Model file for the job. Use its own axes, mm. Face numbers are marked on the shaded views. A direction names the side the tool comes from. Round coordinates to 2 decimals unless told otherwise and drop trailing zeros. Loops run counter-clockwise (first coordinate to the right, second up) from the corner with the lowest first, then second, coordinate; pieces in that order, holes last. Notation, with made-up numbers: (9.5, -40) -> (45.5, -40) arc R29 ccw to (45.5, -9) -> close; hole circle Ø3 at (7, 78.5). An arc over 180 degrees is marked (long way). Use a Markdown table: item, result.
from build123d import *

# Parameters (mm, degrees)
SKETCH2_W           = 25
SKETCH2_H           = 25
BOSS_EXTRUDE1_DEPTH = 20
SKETCH3_W           = 18.8
SKETCH3_H           = 18.8
CUT_EXTRUDE1_DEPTH  = 18.8


with BuildPart() as part:
    # Sketch2 → Boss-Extrude1 (new body)
    with BuildSketch(Plane(origin=(0, 0, 0), x_dir=(1, 0, 0), z_dir=(0, 1, 0))):
        Rectangle(SKETCH2_W, SKETCH2_H)
    extrude(amount=BOSS_EXTRUDE1_DEPTH)

    # Sketch3 → Cut-Extrude1 (cut)
    with BuildSketch(Plane.XZ):
        Rectangle(SKETCH3_W, SKETCH3_H)
    extrude(amount=-CUT_EXTRUDE1_DEPTH, mode=Mode.SUBTRACT)

    # Loft1: read off the stored shape, not the designer's step
    # Loft1: loft between two sections, ruled curve by curve
    loft1_from = [
        Edge.make_bspline([(-12.5, 20, 12.5), (-11.458333333, 20, 12.5), (-10.416666667, 20, 12.5), (-8.333333333, 20, 12.5), (-7.291666667, 20, 12.5), (-5.208333333, 20, 12.5), (-4.166666667, 20, 12.5), (-2.083333333, 20, 12.5), (-1.041666667, 20, 12.5), (1.041666667, 20, 12.5), (2.083333333, 20, 12.5), (4.166666667, 20, 12.5), (5.208333333, 20, 12.5), (7.291666667, 20, 12.5), (8.333333333, 20, 12.5), (10.416666667, 20, 12.5), (11.458333333, 20, 12.5), (12.5, 20, 12.5)], [0, 0, 0, 0, 0.125, 0.125, 0.25, 0.25, 0.375, 0.375, 0.5, 0.5, 0.625, 0.625, 0.75, 0.75, 0.875, 0.875, 1, 1, 1, 1], 3),
        Edge.make_bspline([(12.5, 20, 12.5), (12.5, 20, 11.458333333), (12.5, 20, 10.416666667), (12.5, 20, 8.333333333), (12.5, 20, 7.291666667), (12.5, 20, 5.208333333), (12.5, 20, 4.166666667), (12.5, 20, 2.083333333), (12.5, 20, 1.041666667), (12.5, 20, -1.041666667), (12.5, 20, -2.083333333), (12.5, 20, -4.166666667), (12.5, 20, -5.208333333), (12.5, 20, -7.291666667), (12.5, 20, -8.333333333), (12.5, 20, -10.416666667), (12.5, 20, -11.458333333), (12.5, 20, -12.5)], [0, 0, 0, 0, 0.125, 0.125, 0.25, 0.25, 0.375, 0.375, 0.5, 0.5, 0.625, 0.625, 0.75, 0.75, 0.875, 0.875, 1, 1, 1, 1], 3),
        Edge.make_bspline([(-12.5, 20, -12.5), (-12.5, 20, -11.458333333), (-12.5, 20, -10.416666667), (-12.5, 20, -8.333333333), (-12.5, 20, -7.291666667), (-12.5, 20, -5.208333333), (-12.5, 20, -4.166666667), (-12.5, 20, -2.083333333), (-12.5, 20, -1.041666667), (-12.5, 20, 1.041666667), (-12.5, 20, 2.083333333), (-12.5, 20, 4.166666667), (-12.5, 20, 5.208333333), (-12.5, 20, 7.291666667), (-12.5, 20, 8.333333333), (-12.5, 20, 10.416666667), (-12.5, 20, 11.458333333), (-12.5, 20, 12.5)], [0, 0, 0, 0, 0.125, 0.125, 0.25, 0.25, 0.375, 0.375, 0.5, 0.5, 0.625, 0.625, 0.75, 0.75, 0.875, 0.875, 1, 1, 1, 1], 3),
        Edge.make_bspline([(12.5, 20, -12.5), (11.458333333, 20, -12.5), (10.416666667, 20, -12.5), (8.333333333, 20, -12.5), (7.291666667, 20, -12.5), (5.208333333, 20, -12.5), (4.166666667, 20, -12.5), (2.083333333, 20, -12.5), (1.041666667, 20, -12.5), (-1.041666667, 20, -12.5), (-2.083333333, 20, -12.5), (-4.166666667, 20, -12.5), (-5.208333333, 20, -12.5), (-7.291666667, 20, -12.5), (-8.333333333, 20, -12.5), (-10.416666667, 20, -12.5), (-11.458333333, 20, -12.5), (-12.5, 20, -12.5)], [0, 0, 0, 0, 0.125, 0.125, 0.25, 0.25, 0.375, 0.375, 0.5, 0.5, 0.625, 0.625, 0.75, 0.75, 0.875, 0.875, 1, 1, 1, 1], 3),
    ]
    loft1_to = [
        Edge.make_bspline([(-7.071067812, 30, 7.071067812), (-6.654401145, 30, 7.487734479), (-6.18511191, 30, 7.882942296), (-5.147579804, 30, 8.596441749), (-4.57928395, 30, 8.914502371), (-3.364263, 30, 9.440335189), (-2.717633031, 30, 9.647849649), (-1.380556459, 30, 9.927768934), (-0.690355937, 30, 10), (0.690355937, 30, 10), (1.380556459, 30, 9.927768934), (2.717633031, 30, 9.647849649), (3.364263, 30, 9.440335189), (4.57928395, 30, 8.914502371), (5.147579804, 30, 8.596441749), (6.18511191, 30, 7.882942296), (6.654401145, 30, 7.487734479), (7.071067812, 30, 7.071067812)], [0, 0, 0, 0, 0.125, 0.125, 0.25, 0.25, 0.375, 0.375, 0.5, 0.5, 0.625, 0.625, 0.75, 0.75, 0.875, 0.875, 1, 1, 1, 1], 3),
        Edge.make_bspline([(7.071067812, 30, 7.071067812), (7.487734479, 30, 6.654401145), (7.882942296, 30, 6.18511191), (8.596441749, 30, 5.147579804), (8.914502371, 30, 4.57928395), (9.440335189, 30, 3.364263), (9.647849649, 30, 2.717633031), (9.927768934, 30, 1.380556459), (10, 30, 0.690355937), (10, 30, -0.690355937), (9.927768934, 30, -1.380556459), (9.647849649, 30, -2.717633031), (9.440335189, 30, -3.364263), (8.914502371, 30, -4.57928395), (8.596441749, 30, -5.147579804), (7.882942296, 30, -6.18511191), (7.487734479, 30, -6.654401145), (7.071067812, 30, -7.071067812)], [0, 0, 0, 0, 0.125, 0.125, 0.25, 0.25, 0.375, 0.375, 0.5, 0.5, 0.625, 0.625, 0.75, 0.75, 0.875, 0.875, 1, 1, 1, 1], 3),
        Edge.make_bspline([(-7.071067812, 30, -7.071067812), (-7.487734479, 30, -6.654401145), (-7.882942296, 30, -6.18511191), (-8.596441749, 30, -5.147579804), (-8.914502371, 30, -4.57928395), (-9.440335189, 30, -3.364263), (-9.647849649, 30, -2.717633031), (-9.927768934, 30, -1.380556459), (-10, 30, -0.690355937), (-10, 30, 0.690355937), (-9.927768934, 30, 1.380556459), (-9.647849649, 30, 2.717633031), (-9.440335189, 30, 3.364263), (-8.914502371, 30, 4.57928395), (-8.596441749, 30, 5.147579804), (-7.882942296, 30, 6.18511191), (-7.487734479, 30, 6.654401145), (-7.071067812, 30, 7.071067812)], [0, 0, 0, 0, 0.125, 0.125, 0.25, 0.25, 0.375, 0.375, 0.5, 0.5, 0.625, 0.625, 0.75, 0.75, 0.875, 0.875, 1, 1, 1, 1], 3),
        Edge.make_bspline([(7.071067812, 30, -7.071067812), (6.654401145, 30, -7.487734479), (6.18511191, 30, -7.882942296), (5.147579804, 30, -8.596441749), (4.57928395, 30, -8.914502371), (3.364263, 30, -9.440335189), (2.717633031, 30, -9.647849649), (1.380556459, 30, -9.927768934), (0.690355937, 30, -10), (-0.690355937, 30, -10), (-1.380556459, 30, -9.927768934), (-2.717633031, 30, -9.647849649), (-3.364263, 30, -9.440335189), (-4.57928395, 30, -8.914502371), (-5.147579804, 30, -8.596441749), (-6.18511191, 30, -7.882942296), (-6.654401145, 30, -7.487734479), (-7.071067812, 30, -7.071067812)], [0, 0, 0, 0, 0.125, 0.125, 0.25, 0.25, 0.375, 0.375, 0.5, 0.5, 0.625, 0.625, 0.75, 0.75, 0.875, 0.875, 1, 1, 1, 1], 3),
    ]
    loft1 = Solid(Shell([*[Face.make_surface_from_curves(loft1_from[k], loft1_to[k]) for k in range(4)], Face(Wire(loft1_from)), Face(Wire(loft1_to))]))
    add(loft1)


solid = part.part
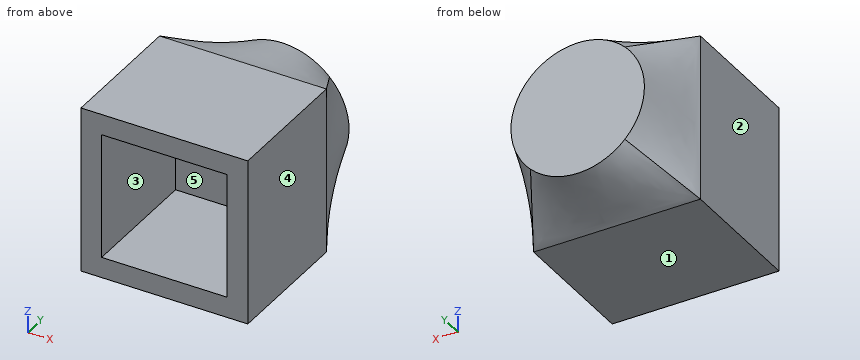
Q1. Tool access for the marked faces 4 and 5: list every direction of +Z, -Z, +X, -X, +Y, -Y with a clear straight run to the whole face (end or side of a thin tool).
Results list:
| item | result |
|---|---|
| face 4 | +Z, -Z, +X, +Y, -Y |
| face 5 | -Y |
Q2. Drill centre lines: L1, parallel to X at y = 16.5, z = -4.75; L2, parallel to Y at x = -4, z = -4.5. Where is each one in solid material? Low to high. Write a range as from..to.
Results list:
| item | result |
|---|---|
| L1 | x = -12.5..-9.4, 9.4..12.5 |
| L2 | y = 18.8..30 |
Q3. Pull direction Z, two halves, no side cores. Call the marked faces 1, 2 and 3: released by +Z, released by -Z, zero draft, split by the parting line, or undercut.
Results list:
| item | result |
|---|---|
| face 1 | released by -Z |
| face 2 | zero draft |
| face 3 | undercut |
Q4. Band-saw the part on A-A, the plane y = 5. Give the cut face in (x, z).
Results list:
| item | result |
|---|---|
| outline | (-12.5, -12.5) -> (12.5, -12.5) -> (12.5, 12.5) -> (-12.5, 12.5) -> close; hole (-9.4, -9.4) -> (9.4, -9.4) -> (9.4, 9.4) -> (-9.4, 9.4) -> close |
Q5. Flat gauge pins, fed straight in: pin 1 (4 mm diameter, centred on x = -7, z = -6, fed in from -Y); pin 2 (10 mm diameter, centred on x = -1, y = 26.5, fed in from -Z). Where does each tip first touch, or does it go through?
Results list:
| item | result |
|---|---|
| pin 1 | stops at y = 18.8 |
| pin 2 | stops at z = -12.12 |
